Could you check a few things on this drawing? It's one solid part, dimensions in mm from its lowest x, y, z. Give positions to 0.01 mm unless a question says otherwise; leave off trailing zeros. Loops run counter-clockwise (first coordinate to the right, second up) from the corner with the lowest first, then second, coordinate; pieces in that order, holes last.
1. For P1, Ø1.5, axis at y = 12, z = 3, coming from the -X side, with a flat end and sliding along its axis, tell me the tip position at first contact or that it passes through.
2. Imagine slicing it at B-B (y = 18.25). List the corners of the cut face in (x, z) for me.
3. Imagine slicing it at A-A (z = 2.35). List the corners of the cut face in (x, y) for me, plus the area to 3 significant figures.
4. I need wall thicknesses on line 1 along X through (y, z) = (3.75, 3.5). Which ranges of the line are inside material? Lowest first, please.
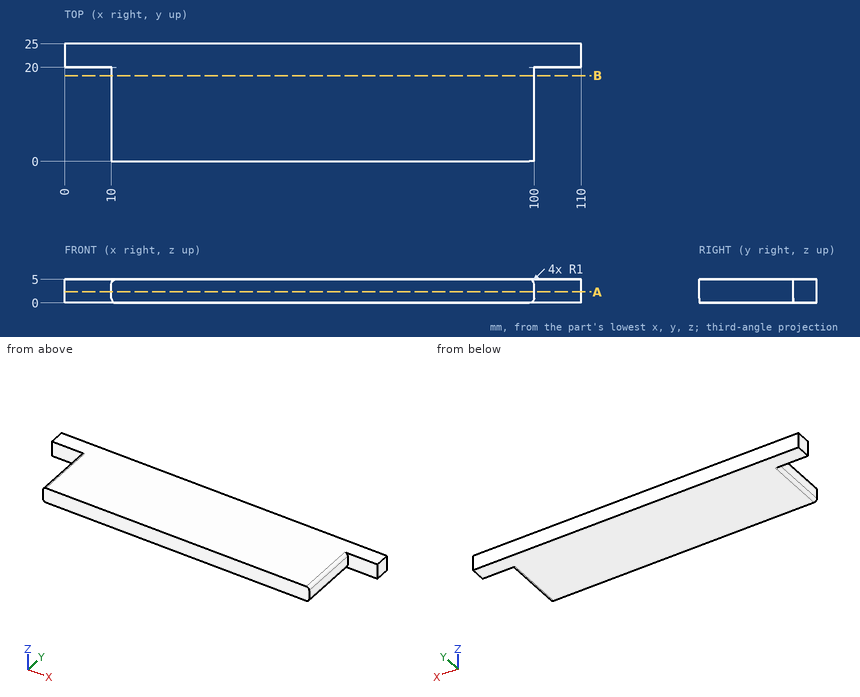
Derived:
1. P1: stops at x = 10
2. outline: (10, 1) arc R1 ccw to (11, 0) - (99, 0) arc R1 ccw to (100, 1) - (100, 4) arc R1 ccw to (99, 5) - (11, 5) arc R1 ccw to (10, 4) - close
3. outline: (0, 20) - (10, 20) - (10, 0) - (100, 0) - (100, 20) - (110, 20) - (110, 25) - (0, 25) - close
3. area: 2,350 mm2
4. line 1: x = 10 to 100
